Autodesk Inventor part; units mm, degrees
ref_plane "YZ Plane" through (0, 0, 0) normal (1, 0, 0) x (0, 1, 0)
ref_plane "XZ Plane" through (0, 0, 0) normal (0, 1, 0) x (-1, 0, 0)
ref_plane "XY Plane" through (0, 0, 0) normal (0, 0, 1) x (1, 0, 0)
sketch "Sketch1" plane through (0, 0, 0) normal (0, 1, 0) x (-1, 0, 0)
  line L0 (0, 0) -> (38.1, 0)
  line L1 (38.1, 0) -> (38.1, -50.8)
  line L2 (38.1, -50.8) -> (0, -50.8)
  line L3 (0, -50.8) -> (0, 0)
  line L4 (38.1, -50.8) -> (33.02, -50.8)
  line L5 (33.02, -50.8) -> (33.02, 0)
  line L6 (33.02, 0) -> (38.1, 0)
  line L7 (38.1, 0) -> (38.1, -50.8)
  line L8 (0, -50.8) -> (5.08, -50.8)
  line L9 (5.08, -50.8) -> (5.08, 0)
  line L10 (5.08, 0) -> (0, 0)
  line L11 (0, 0) -> (0, -50.8)
  dimension "d0" = 38.1
  dimension "d1" = 50.8
  dimension "d2" = 5.08
  dimension "d3" = 5.08
extrude "Extrusion1" add sketch "Sketch1" along normal blind 25.4 contours L0 L9 L2 L3 | L0 L1 L2 L5
extrude "Extrusion2" add sketch "Sketch1" against normal blind 5.08
sketch "Sketch2" plane through (0, 25.4, 0) normal (1, 0, 0) x (0, 0, -1)
  line L0 (50.8, 0) -> (0, 0)
  line L1 (25.4, 0) -> (25.4, -12.7)
  point P0 (0, -25.4)
  dimension "d8" = 12.7
hole "Hole1" at (0, 12.7, -25.4) direction (-1, 0, 0) diameter 6.7564 end through all
sketch "Sketch3" plane through (0, -5.08, 0) normal (0, -1, 0) x (1, 0, 0)
  line L0 (0, 0) -> (-19.05, 0)
  line L1 (0, 0) -> (-38.1, 0)
  line L2 (-19.05, 0) -> (-19.05, -25.4)
  line L3 (-6, -34.85) -> (-6, -15.95)
  line L4 (-6, -15.95) -> (-32.1, -15.95)
  line L5 (-32.1, -15.95) -> (-32.1, -34.85)
  line L6 (-32.1, -34.85) -> (-6, -34.85)
  line L7 (-6, -34.85) -> (-32.1, -15.95) construction
  line L8 (-6, -15.95) -> (-32.1, -34.85) construction
  line L9 (-10, -19.95) -> (-10, -30.85)
  line L10 (-10, -30.85) -> (-28.1, -30.85)
  line L11 (-28.1, -30.85) -> (-28.1, -19.95)
  line L12 (-28.1, -19.95) -> (-10, -19.95)
  line L13 (-10, -19.95) -> (-28.1, -30.85) construction
  line L14 (-10, -30.85) -> (-28.1, -19.95) construction
  dimension "d16" = 25.4
  dimension "d17" = 18.9
  dimension "d18" = 26.1
  dimension "d19" = 10.9
  dimension "d20" = 18.1
extrude "Extrusion3" add sketch "Sketch3" along normal blind 69.85
sketch "Sketch4" plane through (-6, -5.08, -15.95) normal (1, 0, 0) x (0, 0, -1)
  line L0 (18.9, 0) -> (18.9, -69.85)
  line L1 (18.9, -34.925) -> (9.4512, -34.925)
  line L2 (9.4512, -34.925) -> (9.4512, -9.525) construction
  line L3 (12.6262, -34.925) -> (12.6262, -9.525)
  line L4 (6.2762, -9.525) -> (6.2762, -34.925)
  arc A0 (6.2762, -34.925) -> (12.6262, -34.925) centre (9.4512, -34.925) ccw
  arc A1 (12.6262, -9.525) -> (6.2762, -9.525) centre (9.4512, -9.525) ccw
  point P0 (-15.95, 5.08)
  point P1 (9.4512, -22.225)
  dimension "d23" = 9.4488
  dimension "d24" = 25.4
  dimension "d25" = 6.35
extrude "Extrusion4" cut sketch "Sketch4" against normal blind 76.2
fillet "Fillet1" radius 2.54 24 edges at (-38.1, -5.08, -25.4) (0, -5.08, -25.4) (-6, -11.43, -25.4012) (-6, -27.305, -28.5762) (-6, -43.18, -25.4012) (-6, -27.305, -22.2262) (-6, -40.005, -15.95) (-6, -40.005, -34.85) (-6, -74.93, -25.4) (-19.05, -74.93, -15.95) (-19.05, -74.93, -34.85) (-32.1, -74.93, -25.4) (-32.1, -40.005, -15.95) (-32.1, -40.005, -34.85) (-32.1, -27.305, -28.5762) (-32.1, -11.43, -25.4012) (-32.1, -27.305, -22.2262) (-32.1, -43.18, -25.4012) (-19.05, -5.08, -50.8) (-38.1, 10.16, -50.8) (-38.1, 10.16, 0) (-19.05, -5.08, 0) (0, 10.16, -50.8) (0, 10.16, 0)
properties part number "Sample Holder end for 8020-neutron-whispervalve-r2"
Input: part model. Units: mm. Frame: model coordinates. A direction names the side the tool comes from. Coordinates: 2 decimals unless noted, no trailing zeros. Order: outer loops, then holes, each group sorted by start corner. A loop starts at its lowest first (then second) coordinate and runs counter-clockwise, first axis right, second up. Notation, with made-up numbers: M 78.25,8.5 L 127.25,8.5 A15 ccw 127.25,37.5 Z; hole C 86,20.5 d2. An arc over 180 degrees is marked long. Write item = value, one per line. Start each with the question number.
(1) First-contact query: P1, Ø2, axis at x = -5.5, z = -17.5, coming from the -Y side; P2, Ø10, axis at y = -23, z = -30.5, coming from the +X side; P3, Ø20, axis at x = -23, y = -55, coming from the +Z side. Flat tips, straight axial feed; report the tip coordinate or a pass-through.
(2) Pull-direction query (Y, two-part tool) for faces 1 (the flat face through (-18.8, -5.08, -35.2)), 2 (the cylindrical face through (-6.764, -27.127, -29.301)), 3 (the cylindrical face through (-37.336, 11.234, -0.724)); classes: released by +Y, released by -Y, zero draft, split by the parting line, or undercut.
(3) Section B-B on x = -27. Output: boundary loops of the cut face in (y, z), and give its area (3 significant figures).
(4) Section A-A on y = -36.5. Output: boundary loops of the cut face in (x, z).
(5) Reachability of faces 4 (the flat face through (-19, -40, -19.95)), 5 (the cylindrical face through (-28.82, -43.18, -25.33)), 6 (the cylindrical face through (-31.376, -39.206, -34.086)), 7 (the flat face through (-19, -38, -15.95)), 8 (the flat face through (-5.08, 13, -20)) from +Z, -Z, +X, -X, +Y, -Y: full face, straight path, thin tool, end or side. Return the list, or none.
(6) Section D-D on z = -25.4. Give the number of separate pieces and of enclosed holes in the cut face, and give its area (3 significant figures).
(7) Section C-C on y = 12.7. Output: boundary loops of the cut face in (x, z).
(8) Line query: line 1 along Y through (x, z) = (-34.9, -25.4); line 2 along Z through (x, y) = (-35.2, 12.7); line 3 along X through (y, z) = (2, -43). Output: solid intervals per line, ascending. Write a range as [from, to].
Result set:
q1.P1 = -73.66
q1.P2 = -6
q1.P3 = -15.95
q2.face_1 = released by -Y
q2.face_2 = undercut
q2.face_3 = zero draft
q3.outline = M -74.93,-32.31 A2.54 ccw -72.39,-34.85 L -5.08,-34.85 L -5.08,-48.26 A2.54 ccw -2.54,-50.8 L 0,-50.8 L 0,0 L -2.54,0 A2.54 ccw -5.08,-2.54 L -5.08,-15.95 L -72.39,-15.95 A2.54 ccw -74.93,-18.49 L -74.93,-19.95 L -5.08,-19.95 L -5.08,-30.85 L -74.93,-30.85 Z
q3.area = 811 mm²
q4.outline = M -32.1,-32.31 A2.54 ccw -29.56,-34.85 L -8.54,-34.85 A2.54 ccw -6,-32.31 L -6,-31.12 A2.54 ccw -8.54,-28.58 L -10,-28.58 L -10,-30.85 L -28.1,-30.85 L -28.1,-28.58 L -29.56,-28.58 A2.54 ccw -32.1,-31.12 Z; M -32.1,-19.69 A2.54 ccw -29.56,-22.23 L -28.1,-22.23 L -28.1,-19.95 L -10,-19.95 L -10,-22.23 L -8.54,-22.23 A2.54 ccw -6,-19.69 L -6,-18.49 A2.54 ccw -8.54,-15.95 L -29.56,-15.95 A2.54 ccw -32.1,-18.49 Z
q5.face_4 = -Y
q5.face_5 = +X, -X
q5.face_6 = -Z, -X, -Y
q5.face_7 = +Z, +X, -X, -Y
q5.face_8 = +Z, -Z, +Y
q6.separate_pieces = 5
q6.enclosed_holes = 0
q6.area = 677 mm²
q7.outline = M -38.1,-48.26 A2.54 ccw -35.56,-50.8 L -33.02,-50.8 L -33.02,-28.78 L -38.1,-28.78 Z; M -38.1,-22.02 L -33.02,-22.02 L -33.02,0 L -35.56,0 A2.54 ccw -38.1,-2.54 Z; M -5.08,-50.8 L -2.54,-50.8 A2.54 ccw 0,-48.26 L 0,-28.78 L -5.08,-28.78 Z; M -5.08,-22.02 L 0,-22.02 L 0,-2.54 A2.54 ccw -2.54,0 L -5.08,0 Z
q8.line_1 = [-5.08, 9.32], [16.08, 25.4]
q8.line_2 = [-50.8, -28.78], [-22.02, 0]
q8.line_3 = [-38.1, -33.02], [-5.08, 0]
